Can you work these out from the model? Positions are in its coordinate system, mm. A direction names the side the tool comes from. Round coordinates to 2 decimals unless told otherwise and drop trailing zeros. Write each loop counter-clockwise with the first axis right and the second up, starting at its lowest first coordinate (ties: lowest second). Pieces come first, ordered by that corner, then holes. Notation, with made-up numbers: M 42.5,22 L 67.5,22 A25 cw 67.5,42 Z; hole C -36,-12 d10. An arc over 180 degrees is marked long. Answer as a JSON object with one key per item and string values. Group by question number.
1) Please list where these lines run through material, in increasing order: L1, parallel to Y at x = -10.5, z = 4; L2, parallel to Y at x = -16, z = 32; L3, parallel to X at y = 38, z = 8. Write a range as [from, to].
2) Suppose I cut it at A-A, the plane z = 38. Write out the boundary of the cut face in (x, y).
3) Suppose I cut it at C-C, the plane x = -19.5. Write out the boundary of the cut face in (y, z).
4) Suppose I cut it at B-B, the plane y = -26. Write out the boundary of the cut face in (x, z), and give its area (3 significant figures).
5) Suppose I cut it at D-D, the plane z = 29. Write out the boundary of the cut face in (x, y).
6) I'm going to push flat-ended pins straight in: pin 1 Ø1 at (x, z) = (11.5, 24) entering from -Y; pin 2 Ø3.5 at (x, y) = (-4.5, -3) entering from +Z; pin 3 Ø8 at (x, y) = (-26.5, 4.5) entering from +Z. Where does each tip first touch, or does it pass through?
7) On a 3-axis mill with a long thin cutter (end or side, diameter ignored), from which of +Z, -Z, +X, -X, +Y, -Y can I reach the whole of each face in a straight line? I mean faces 3 (the flat face through (-30, -10.733, 5)), 4 (the flat face through (-2, -33.593, 16)), 5 (the flat face through (-2, -34.093, 38)). Say none if no direction works.
8) If we mould it in two halves opening along X, with no side actions, what happens to faces 1 (the flat face through (28, -10.733, 5)), 2 (the flat face through (-2, 55.307, 16))? For each: +X half, -X half, draft (parallel to the pull), parting line (faces both ways), or undercut.
from build123d import *

# Parameters (mm, degrees)
F0_W     = 66.675
F0_H     = 88.9
F1_DEPTH = 44.45
F2_T     = -2.54
F4_DEPTH = 5.08
F3_W     = 55.499
F3_H     = 3.175
F5_DEPTH = 3.048
F6_W     = 66.675
F6_H     = 12.7
F7_DEPTH = 0.5
F8_W     = 66.675
F8_H     = 12.6965791702
F9_DEPTH = 0.5


with BuildPart() as f1:
    # F0 (on Top) → F1 (new body)
    with BuildSketch(Plane.XY):
        with Locations((-1.1231470853, 10.8568438743)):
            Rectangle(F0_W, F0_H)
    extrude(amount=F1_DEPTH)

    # F2
    f2_openings = [f1.faces().sort_by_distance(p)[0] for p in [
        (-1.123147, 10.856844, 44.45),
    ]]
    offset(amount=F2_T, openings=f2_openings)

    # F3 (on face) → F4 (join)
    with BuildSketch(Plane.XY.offset(2.54)):
        Polygon((29.6743529147, 40.0668438743), (26.6263529147, 40.0668438743), (26.6263529147, -1.4621561257), (26.6263529147, -4.6371561257), (26.6263529147, -10.7331561257), (29.6743529147, -10.7331561257), align=None)
        Polygon((-28.8726470853, 40.0668438743), (-31.9206470853, 40.0668438743), (-31.9206470853, -10.7331561257), (-28.8726470853, -10.7331561257), (-28.8726470853, -4.6371561257), (-28.8726470853, -1.4621561257), align=None)
    extrude(amount=F4_DEPTH)

    # F3 (on face) → F5 (join)
    with BuildSketch(Plane.XY.offset(2.54)):
        with Locations((-1.1231470853, -3.0496561257)):
            Rectangle(F3_W, F3_H)
    extrude(amount=F5_DEPTH)

    # F6 (on face) → F7 (join)
    with BuildSketch(Plane(origin=(0, 55.3068438743, 0), x_dir=(-1, 0, 0), z_dir=(0, 1, 0))):
        with Locations((1.1231470853, 38.1)):
            Rectangle(F6_W, F6_H)
    extrude(amount=F7_DEPTH)

    # F8 (on face) → F9 (join)
    with BuildSketch(Plane.XZ.offset(33.5931561257)):
        with Locations((-1.1231470853, 38.1017104149)):
            Rectangle(F8_W, F8_H)
    extrude(amount=F9_DEPTH)


solid = f1.part
Results:
{
 "1": {"L1": "[-33.59, -31.05], [-4.64, -1.46], [52.77, 55.31]", "L2": "[-34.09, -31.05], [52.77, 55.81]", "L3": "[-34.46, -31.92], [29.67, 32.21]"},
 "2": {"outline": "M -34.46,-34.09 L 32.21,-34.09 L 32.21,55.81 L -34.46,55.81 Z; hole M -31.92,-31.05 L 29.67,-31.05 L 29.67,52.77 L -31.92,52.77 Z"},
 "3": {"outline": "M -34.09,31.75 L -33.59,31.75 L -33.59,0 L 55.31,0 L 55.31,31.75 L 55.81,31.75 L 55.81,44.45 L 52.77,44.45 L 52.77,2.54 L -1.46,2.54 L -1.46,5.59 L -4.64,5.59 L -4.64,2.54 L -31.05,2.54 L -31.05,44.45 L -34.09,44.45 Z"},
 "4": {"outline": "M -34.46,0 L 32.21,0 L 32.21,44.45 L 29.67,44.45 L 29.67,2.54 L -31.92,2.54 L -31.92,44.45 L -34.46,44.45 Z", "area": "382 mm^2"},
 "5": {"outline": "M -34.46,-33.59 L 32.21,-33.59 L 32.21,55.31 L -34.46,55.31 Z; hole M -31.92,-31.05 L 29.67,-31.05 L 29.67,52.77 L -31.92,52.77 Z"},
 "6": {"pin 1": "y = -33.59", "pin 2": "z = 5.59", "pin 3": "z = 7.62"},
 "7": {"face 3": "+Z", "face 4": "-Z, +X, -X, -Y", "face 5": "+Z, -Z, +X, -X, -Y"},
 "8": {"face 1": "undercut", "face 2": "draft"}
}
